Could you check a few things on this model? Use its own coordinates, in mm. Face numbers are marked on the shaded views. Coordinates: 2 decimals unless noted, no trailing zeros. Loops run counter-clockwise (first coordinate to the right, second up) from the corner with the lowest first, then second, coordinate; pieces in that order, holes last. Notation, with made-up numbers: (-36.75, 34) -> (7.25, 34) arc R28 cw to (7.25, 71) -> close; hole circle Ø8 at (70, 23.25). An arc over 180 degrees is marked (long way). One line per question, with ' | ' between items.
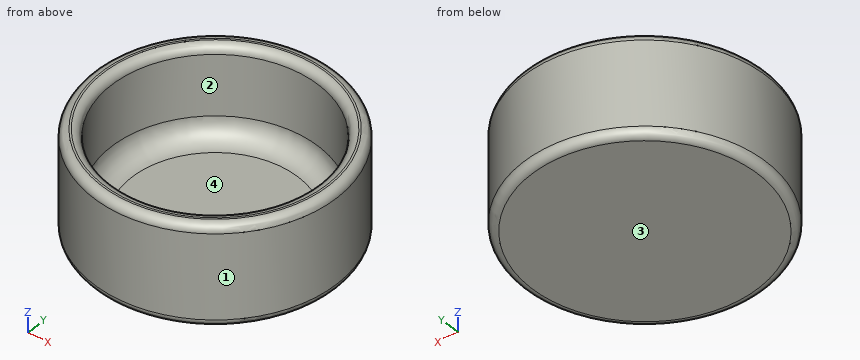
```python
from build123d import *

# Parameters (mm, degrees)
F0_R     = 30
F0_R_2   = 25.55
F1_DEPTH = 3
F2_DEPTH = 25
F3_R     = 5
F4_R     = 2
F0_R_3   = 40
F0_R_4   = 30.5
F5_DEPTH = 27.3
F6_R     = 2


with BuildPart() as f1:
    # F0 (on Top) → F1 (new body)
    with BuildSketch(Plane.XY):
        Circle(F0_R)
        Circle(F0_R_2, mode=Mode.SUBTRACT)
        Circle(F0_R_2)
    extrude(amount=F1_DEPTH)

    # F0 (on Top) → F2 (join)
    with BuildSketch(Plane.XY):
        Circle(F0_R)
        Circle(F0_R_2, mode=Mode.SUBTRACT)
    extrude(amount=F2_DEPTH)

    # F3
    f3_edges = [f1.edges().sort_by_distance(p)[0] for p in [
        (-25.55, 0, 3),
    ]]
    fillet(f3_edges, radius=F3_R)

    # F4
    f4_edges = [f1.edges().sort_by_distance(p)[0] for p in [
        (-25.55, 0, 25),
        (-30, 0, 25),
    ]]
    fillet(f4_edges, radius=F4_R)

    # F0 (on Top) → F5 (cut)
    with BuildSketch(Plane.XY):
        Circle(F0_R_3)
        Circle(F0_R_4, mode=Mode.SUBTRACT)
    extrude(amount=F5_DEPTH, mode=Mode.SUBTRACT)

    # F6
    f6_edges = [f1.edges().sort_by_distance(p)[0] for p in [
        (-30, 0, 0),
    ]]
    fillet(f6_edges, radius=F6_R)


solid = f1.part
```
Q1. Imagine slicing it at A-A on y = 0. Write out the boundary of the cut face in (x, z).
Values follow:
outline: (-30, 2) arc R2 ccw to (-28, 0) -> (28, 0) arc R2 ccw to (30, 2) -> (30, 23) arc R2 ccw to (28, 25) -> (27.55, 25) arc R2 ccw to (25.55, 23) -> (25.55, 8) arc R5 cw to (20.55, 3) -> (-20.55, 3) arc R5 cw to (-25.55, 8) -> (-25.55, 23) arc R2 ccw to (-27.55, 25) -> (-28, 25) arc R2 ccw to (-30, 23) -> close
Q2. For pin 1 (3 mm diameter, centred on x = -4.5, y = 12.5, fed in from +Z); pin 2 (10 mm diameter, centred on y = 8, z = 5.5, fed in from +X); pin 3 (2 mm diameter, centred on x = 5, z = 22, fed in from +Y); pin 4 (1.5 mm diameter, centred on x = 2, y = 5.5, fed in from -Z), each with a flat end and sliding along its axis, tell me the tip position at first contact or that it passes through.
Values follow:
pin 1: stops at z = 3 | pin 2: stops at x = 29.85 | pin 3: stops at y = 29.73 | pin 4: stops at z = 0
Q3. Please list where these lines run through material, in increasing order: L1, parallel to Y at x = 0, z = 19.5; L2, parallel to Z at x = 15, y = -12; L3, parallel to Y at x = -21.5, z = 14.5. Write a range as [from, to].
Values follow:
L1: y = [-30, -25.55], [25.55, 30] | L2: z = [0, 3] | L3: y = [-20.92, -13.8], [13.8, 20.92]
Q4. Imagine slicing it at C-C on z = 14.5. Write out the boundary of the cut face in (x, y), plus the area to 3 significant figures.
Values follow:
outline: circle Ø60 at (0, 0); hole circle Ø51.1 at (0, 0) | area: 777 mm2
Q5. We'd pull the mould along Y, two halves only. Please class the marked faces 1, 2, 3 and 4: released by +Y, released by -Y, zero draft, split by the parting line, or undercut.
Values follow:
face 1: split by the parting line | face 2: undercut | face 3: zero draft | face 4: undercut
Q6. Imagine slicing it at D-D on z = 5.25. Write out the boundary of the cut face in (x, y), plus the area to 3 significant figures.
Values follow:
outline: circle Ø60 at (0, 0); hole circle Ø49.45 at (0, 0) | area: 907 mm2
